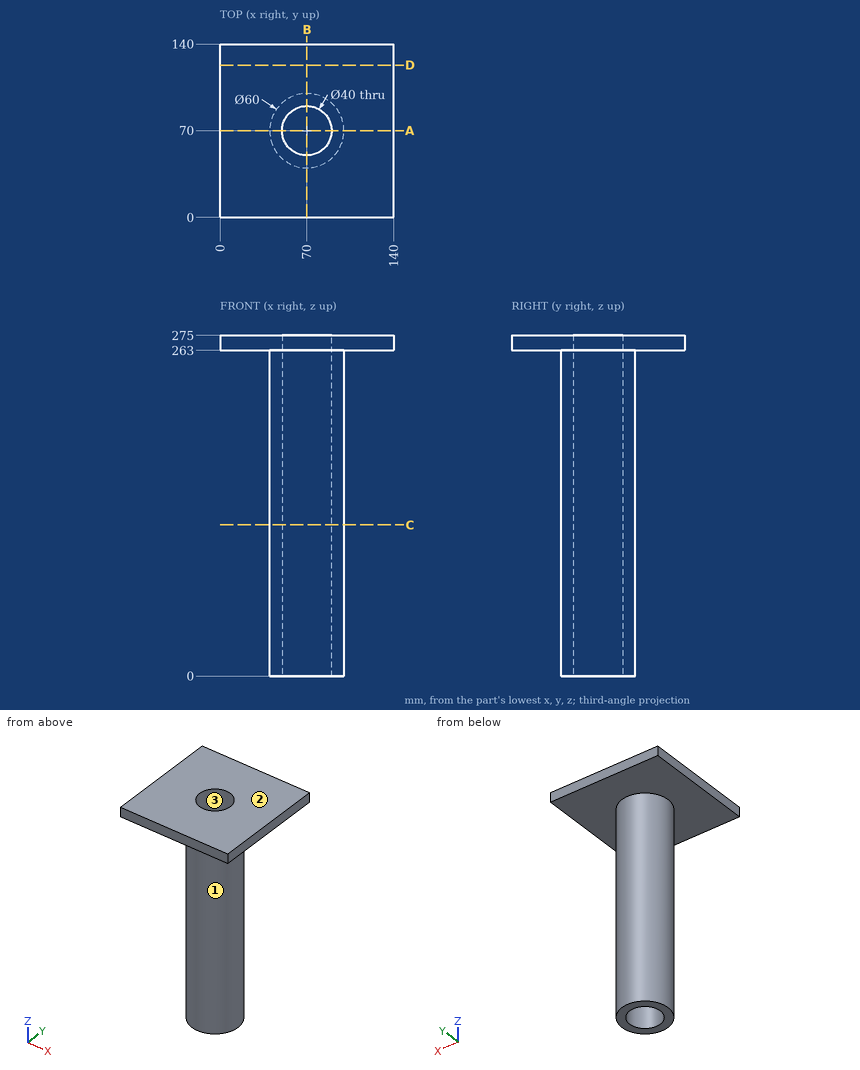
Answer from the drawing. Dimensions are ordinates in mm from the lowest x, y and z of the part. Round coordinates to 2 decimals unless told otherwise and drop trailing zeros. Order: outer loops, then holes, each group sorted by start corner. A loop starts at its lowest first (then second) coordinate and runs counter-clockwise, first axis right, second up.
1) The part is cut by section D-D on y = 123. Write down the section's boundary in (x, z).
2) The part is cut by section C-C on z = 122. Write down the section's boundary in (x, y), plus the area to 3 significant figures.
3) The mould has two halves that part along X. Classify the marked faces 1, 2 and 3: released by +X, released by -X, zero draft, split by the parting line, or undercut.
4) Straight lines are drawn through the part: L1, parallel to Y at x = 70, z = 177.5; L2, parallel to Z at x = 80, y = 106; L3, parallel to Y at x = 55, z = 199.5. For each, find the intervals that lie inside material, in ascending order.
5) The part is cut by section A-A on y = 70. Write down the section's boundary in (x, z).
6) Flat-ended cylindrical pins translate along their axes: pin 1 (12 mm diameter, centred on x = 99, y = 61.5, fed in from -Z); pin 2 (1 mm diameter, centred on y = 87, z = 225, fed in from -X); pin 3 (2 mm diameter, centred on x = 45.5, z = 68.5, fed in from -Y); pin 4 (12 mm diameter, centred on x = 88, z = 104.5, fed in from +Y). Find the tip coordinate at first contact, or state that the pin passes through.
Resolved:
1. outline: (0, 263) - (140, 263) - (140, 275) - (0, 275) - close
2. outline: circle Ø60 at (70, 70); hole circle Ø40 at (70, 70)
2. area: 1,570 mm2
3. face 1: split by the parting line
3. face 2: zero draft
3. face 3: undercut
4. L1: y = 40 to 50, 90 to 100
4. L2: z = 263 to 275
4. L3: y = 44.02 to 56.77, 83.23 to 95.98
5. outline: (0, 263) - (40, 263) - (40, 0) - (50, 0) - (50, 275) - (0, 275) - close; (90, 0) - (100, 0) - (100, 263) - (140, 263) - (140, 275) - (90, 275) - close
6. pin 1: stops at z = 0
6. pin 2: stops at x = 44.95
6. pin 3: stops at y = 51.35
6. pin 4: stops at y = 97.5
